Study the drawing (mm; zero at the part's minimum x, y, z) and answer. A direction names the side the tool comes from. Give positions to 0.01 mm unless a question says otherwise; leave off trailing zeros. Order: outer loops, then holes, each group sorted by start corner. A loop starts at its lowest first (then second) coordinate and runs counter-clockwise, first axis right, second up. Notation, with made-up numbers: (41.5, 6.5) - (79.5, 6.5) arc R13 cw to (79.5, 28.5) - close; hole circle Ø3 at (-23, 51). An arc over 180 degrees is marked (long way). Use CSV: the item, a comma, the result in double quotes.
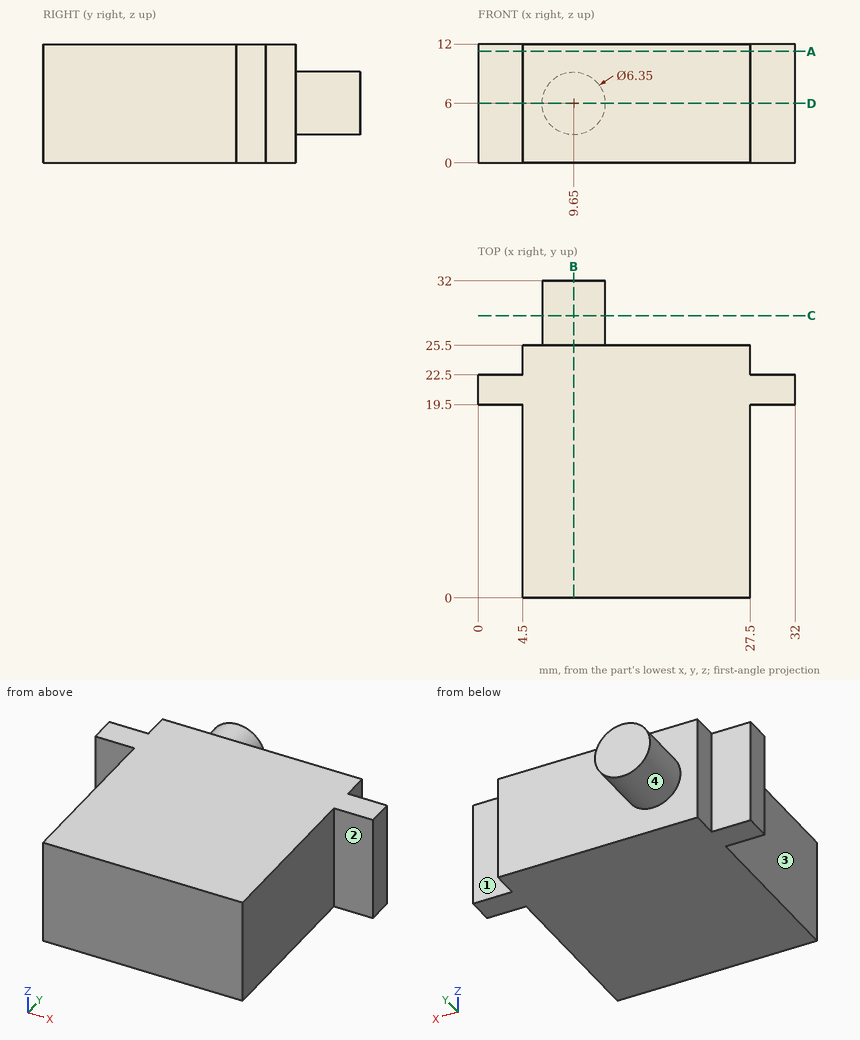
Item 1: The part is cut by section B-B (x = 9.65). Give the vertices of the cut face in (y, z) (3 decimals), and give its area (3 significant figures).
Taken from the geometry:
outline,"(0, 0) - (25.5, 0) - (25.5, 2.825) - (32, 2.825) - (32, 9.175) - (25.5, 9.175) - (25.5, 12) - (0, 12) - close"
area,"347 mm^2"
Item 2: Which of the six approach directions +Z, -Z, +X, -X, +Y, -Y give full straight-line access (tool end or side, diameter ignored) to the marked faces 1, 2, 3 and 4?
Taken from the geometry:
face 1,"+Z, -Z, +X, +Y"
face 2,"+Z, -Z, +X, -Y"
face 3,"+Z, -Z, -X, -Y"
face 4,"+Y"
Item 3: The part is cut by section A-A (z = 11.25). Give the vertices of the cut face in (x, y).
Taken from the geometry:
outline,"(0, 19.5) - (4.5, 19.5) - (4.5, 0) - (27.5, 0) - (27.5, 19.5) - (32, 19.5) - (32, 22.5) - (27.5, 22.5) - (27.5, 25.5) - (4.5, 25.5) - (4.5, 22.5) - (0, 22.5) - close"
Item 4: Find the intervals of material crossed by line 1 along Y through (x, z) = (31.5, 6); line 2 along X through (y, z) = (16, 7.75); line 3 along Y through (x, z) = (5, 1.5), in increasing order.
Taken from the geometry:
line 1,"19.5 to 22.5"
line 2,"4.5 to 27.5"
line 3,"0 to 25.5"
Item 5: Each of these flat-tipped pins is pushed along its axis until it touches: pin 1 (1.3 mm diameter, centred on x = 29.5, z = 7, fed in from -Y); pin 2 (3.5 mm diameter, centred on x = 30.5, z = 8.5, fed in from +Y); pin 3 (1.5 mm diameter, centred on y = 11.5, z = 7, fed in from -X). Where does it stop, or does it pass through?
Taken from the geometry:
pin 1,"y = 19.5"
pin 2,"y = 22.5"
pin 3,"x = 4.5"
Item 6: The part is cut by section D-D (z = 6). Give the vertices of the cut face in (x, y) (3 decimals).
Taken from the geometry:
outline,"(0, 19.5) - (4.5, 19.5) - (4.5, 0) - (27.5, 0) - (27.5, 19.5) - (32, 19.5) - (32, 22.5) - (27.5, 22.5) - (27.5, 25.5) - (12.825, 25.5) - (12.825, 32) - (6.475, 32) - (6.475, 25.5) - (4.5, 25.5) - (4.5, 22.5) - (0, 22.5) - close"
Item 7: The part is cut by section C-C (y = 28.5). Give the vertices of the cut face in (x, z) (3 decimals), and give its area (3 significant figures).
Taken from the geometry:
outline,"circle Ø6.35 at (9.65, 6)"
area,"31.7 mm^2"
